Can you work these out from the drawing? Everything is in mm from the part's minimum corner. A direction names the side the tool comes from. Give positions to 0.01 mm unless a question says otherwise; leave off trailing zeros. Write each loop counter-clockwise with the first axis right and the second up, starting at its lowest first coordinate (ties: lowest second). Pieces come first, ordered by that corner, then holes. Notation, with made-up numbers: (-27.75, 33.25) -> (30.25, 33.25) arc R18 ccw to (30.25, 64.25) -> close; hole circle Ø4 at (-12.5, 7). An arc over 180 degrees is marked (long way). Use one line per item in the form item = value.
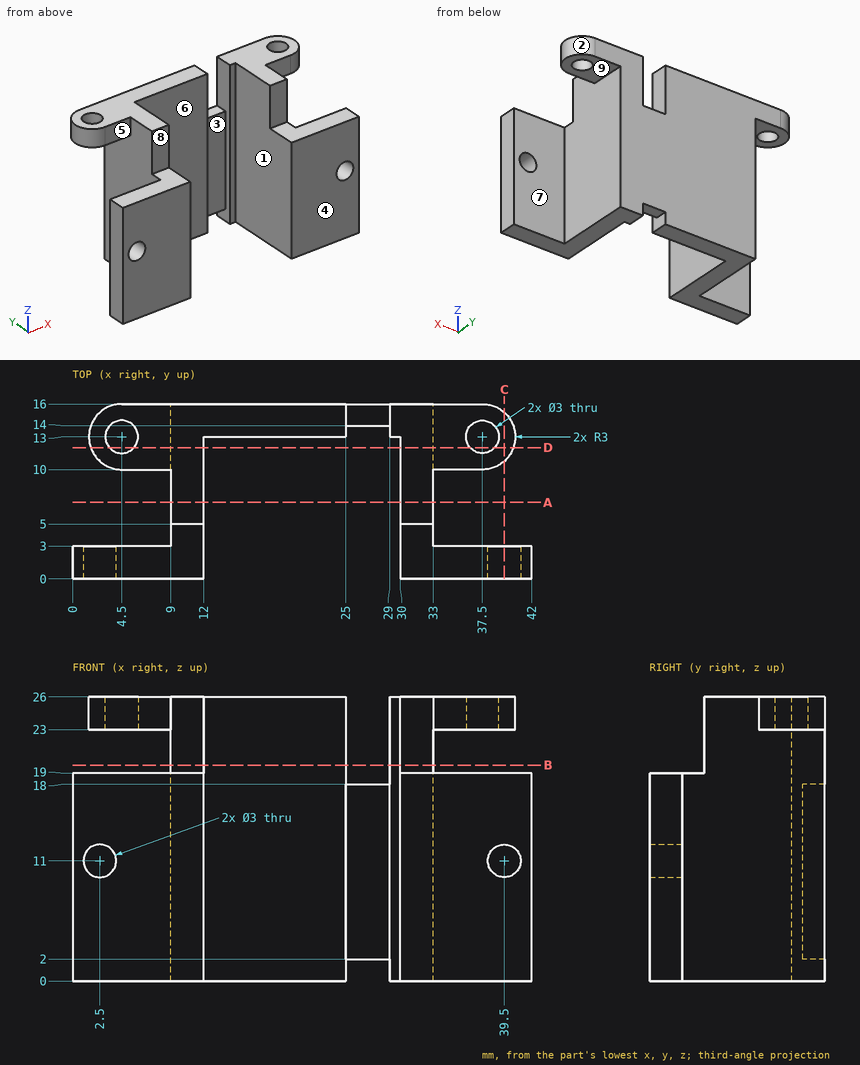
Q1. Which directions (+Z, -Z, +X, -X, +Y, -Y) give clear straight access to the entire face, cutting with the end or side of a thin tool? Please do the marked faces 5, 6, 7, 8 and 9.
Result set:
face_5 = +Z, -Z, -X, -Y
face_6 = +Z, -Z, -Y
face_7 = +Z, -Z, +X, +Y
face_8 = +Z, +X, -X, -Y
face_9 = -Z, +X, +Y, -Y
Q2. Will these pins go through, and if not, where does the flat tip stop? pin 1 Ø4 at (y, z) = (11, 14) entering from +X; pin 2 Ø10.5 at (x, z) = (21, 18) entering from -Y; pin 3 Ø2.5 at (x, z) = (10.5, 21.5) entering from -Y; pin 4 Ø2.5 at (x, y) = (37.5, 13) entering from -Z.
Result set:
pin_1 = 33
pin_2 = 13
pin_3 = 5
pin_4 = through
Q3. I want a section at C-C, the plane x = 39.5. Write out the boundary of the cut face in (y, z).
Result set:
outline = (0, 0) -> (3, 0) -> (3, 9.5) -> (0, 9.5) -> close; (0, 12.5) -> (3, 12.5) -> (3, 19) -> (0, 19) -> close; (10.76, 23) -> (15.24, 23) -> (15.24, 26) -> (10.76, 26) -> close
Q4. If I drill on line 1 along X through (y, z) = (2.15, 11); line 2 along Y through (x, z) = (37.5, 24.7); line 3 along Z through (x, y) = (2.5, 1.8), over which ranges is the centre line in solid material (lowest first)? Write a range as from..to.
Result set:
line_1 = 0..1, 4..12, 30..38, 41..42
line_2 = 10..11.5, 14.5..16
line_3 = 0..9.5, 12.5..19
Q5. I want a section at B-B, the plane z = 19.75. Write out the boundary of the cut face in (x, y).
Result set:
outline = (9, 5) -> (12, 5) -> (12, 13) -> (25, 13) -> (25, 16) -> (9, 16) -> close; (29, 13) -> (30, 13) -> (30, 5) -> (33, 5) -> (33, 16) -> (29, 16) -> close
Q6. If we mould it in two halves opening along X, with no side actions, what happens to the marked faces 1, 2, 3 and 4? For each: +X half, -X half, draft (parallel to the pull), parting line (faces both ways), or undercut.
Result set:
face_1 = undercut
face_2 = +X half
face_3 = undercut
face_4 = draft
Q7. I want a section at A-A, the plane y = 7. Write out the boundary of the cut face in (x, z).
Result set:
outline = (9, 0) -> (12, 0) -> (12, 26) -> (9, 26) -> close; (30, 0) -> (33, 0) -> (33, 26) -> (30, 26) -> close
Q8. I want a section at D-D, the plane y = 12. Write out the boundary of the cut face in (x, z), and give its area (3 significant figures).
Result set:
outline = (1.67, 23) -> (3.38, 23) -> (3.38, 26) -> (1.67, 26) -> close; (5.62, 23) -> (9, 23) -> (9, 0) -> (12, 0) -> (12, 26) -> (5.62, 26) -> close; (30, 0) -> (33, 0) -> (33, 23) -> (36.38, 23) -> (36.38, 26) -> (30, 26) -> close; (38.62, 23) -> (40.33, 23) -> (40.33, 26) -> (38.62, 26) -> close
area = 187 mm2
